from build123d import *

# Parameters (mm, degrees)
SKETCH2_R             = 6.35
BOSS_EXTRUDE1_DEPTH   = 19.05
BOSS_EXTRUDE1_2_DEPTH = 19.05
SKETCH3_W             = 139.7
SKETCH3_H             = 31.75
BOSS_EXTRUDE2_DEPTH   = 6.35
BOSS_EXTRUDE3_REACH   = 75.737
SKETCH9_W             = 133.75
SKETCH9_H             = 25.8
CUT_EXTRUDE1_DEPTH    = 3.175
CHAMFER2_SIZE         = 1.5875
HOLE1_D               = 5.715
HOLE1_DEPTH           = 12.7
HOLE1_CBORE_D         = 6.604
HOLE1_CBORE_DEPTH     = 0.6858


with BuildPart() as part:
    # Sketch2 → Boss-Extrude1 (new body)
    with BuildSketch(Plane(origin=(0, 0, 0), x_dir=(1, 0, 0), z_dir=(0, 1, 0))):
        with Locations(Location((-50.8, 0, 0), (0, 0, 90))):
            Circle(SKETCH2_R)
    extrude(amount=BOSS_EXTRUDE1_DEPTH)



with BuildPart() as body_2:
    # Sketch2 → Boss-Extrude1 2 (new body)
    with BuildSketch(Plane(origin=(0, 0, 0), x_dir=(1, 0, 0), z_dir=(0, 1, 0))):
        with Locations(Location((50.8, 0, 0), (0, 0, 90))):
            Circle(SKETCH2_R)
    extrude(amount=BOSS_EXTRUDE1_2_DEPTH)


with BuildPart() as part_1:
    add(part.part)

    add(body_2.part)  # Boss-Extrude2 merges body 2
    # Sketch3 → Boss-Extrude2 (add)
    with BuildSketch(Plane(origin=(0, 5.650833475, 8.701520484), x_dir=(-1, 0, 0), z_dir=(0, 0.5446390350150281, 0.8386705679454234))):
        with Locations((0, -15.976674319)):
            Rectangle(SKETCH3_W, SKETCH3_H)
    extrude(amount=BOSS_EXTRUDE2_DEPTH)

    # Sketch8 → Boss-Extrude3 (add, up to next)
    with BuildSketch(Plane(origin=(0, 19.05, 0), x_dir=(1, 0, 0), z_dir=(0, 1, 0)), mode=Mode.PRIVATE) as boss_extrude3_sk1:
        with BuildLine():
            Line((44.45, 0), (57.15, 0))
            ThreePointArc((57.15, 0), (50.8, 6.35), (44.45, 0))
        make_face()
    boss_extrude3_tool1 = extrude(boss_extrude3_sk1.sketch, amount=BOSS_EXTRUDE3_REACH, mode=Mode.PRIVATE) - part_1.part
    # Sketch8 → Boss-Extrude3 (add, up to next)
    with BuildSketch(Plane(origin=(0, 19.05, 0), x_dir=(1, 0, 0), z_dir=(0, 1, 0)), mode=Mode.PRIVATE) as boss_extrude3_sk2:
        with BuildLine():
            ThreePointArc((-44.45, 0), (-50.8, 6.35), (-57.15, 0))
            Line((-57.15, 0), (-44.45, 0))
        make_face()
    boss_extrude3_tool2 = extrude(boss_extrude3_sk2.sketch, amount=BOSS_EXTRUDE3_REACH, mode=Mode.PRIVATE) - part_1.part
    add(boss_extrude3_tool1.solids().sort_by_distance((50.8, 19.05, -2.695024))[0])
    add(boss_extrude3_tool2.solids().sort_by_distance((-50.8, 19.05, -2.695024))[0])

    # Sketch9 → Cut-Extrude1 (cut)
    with BuildSketch(Plane(origin=(0, 9.109291347, 14.02707859), x_dir=(1, 0, 0), z_dir=(0, 0.5446390350150282, 0.8386705679454234))):
        with Locations((0, 15.976674319)):
            Rectangle(SKETCH9_W, SKETCH9_H)
    extrude(amount=-CUT_EXTRUDE1_DEPTH, mode=Mode.SUBTRACT)

    # Chamfer2
    chamfer2_edges = [part_1.edges().sort_by_distance(p)[0] for p in [
        (69.85, 19.05, 0),
        (0, 5.736104734, 8.646144681),
        (0, 32.363895266, -8.646144681),
        (69.85, 34.093124202, -5.983365628),
        (-69.85, 19.05, 0),
        (-69.85, 34.093124202, -5.983365628),
        (0, 9.194562606, 13.971702787),
        (-69.85, 7.46533367, 11.308923734),
        (69.85, 22.508457872, 5.325558106),
        (69.85, 7.46533367, 11.308923734),
        (0, 35.822353138, -3.320586574),
        (-69.85, 22.508457872, 5.325558106),
    ]]
    chamfer(chamfer2_edges, length=CHAMFER2_SIZE)

    # Hole1
    with Locations(Plane(origin=(-50.8, 0, 0), x_dir=(0, 0, -1), z_dir=(0, -1, 0))):
        with Locations((0, 0), (0, 101.6)):
            CounterBoreHole(HOLE1_D / 2, HOLE1_CBORE_D / 2, HOLE1_CBORE_DEPTH, depth=HOLE1_DEPTH)


solid = part_1.part
The model under review builds one solid part; all positions refer to its coordinate system, in mm. A direction names the side the tool comes from. Round coordinates to 2 decimals unless told otherwise and drop trailing zeros. Order: outer loops, then holes, each group sorted by start corner. A loop starts at its lowest first (then second) coordinate and runs counter-clockwise, first axis right, second up. Notation, with made-up numbers: (-31.75, -11) -> (-4.75, -11) arc R24 ccw to (-4.75, 2) -> close; hole circle Ø9 at (-3, -24.75). An arc over 180 degrees is marked (long way). Return JSON: item names as keys, results as strings.
1. For L1, parallel to X at y = 0.25, z = 0; L2, parallel to X at y = 7.25, z = 0; L3, parallel to X at y = 28, z = 1.25 (3 decimals), list the stretches that pass through material, from the lowest coordinate up. Write a range as [from, to].
Answer block:
{"L1": "x = [-57.15, -54.1], [-47.5, -44.45], [44.45, 47.5], [54.1, 57.15]", "L2": "x = [-57.15, -53.66], [-47.94, -44.45], [44.45, 47.94], [53.66, 57.15]", "L3": "x = [-68.69, -66.875], [66.875, 68.69]"}
2. The part is to be moulded in two halves that separate along X. For faces 1 (the face through (-69.85, 21, 3)), 2 (the face through (0.956, 9.443, 12.877)), 3 (the face through (51, 12.7, 0)), say which applies: +X half, -X half, draft (parallel to the pull), parting line (faces both ways), or undercut.
Answer block:
{"face 1": "-X half", "face 2": "draft", "face 3": "undercut"}
3. Insertion check: P1, Ø3, axis at x = -0.5, z = 3.5, coming from the -Y side; P2, Ø1.5, axis at x = 25, z = -2, coming from the +Y side; P3, Ø3.5, axis at x = 50.8, z = 0, coming from the +Y side. Each pin has a flat end and moves straight along its axis. Give the tip position at first contact, or say it passes through.
Answer block:
{"P1": "stops at y = 11.35", "P2": "stops at y = 34.55", "P3": "stops at y = 33.4"}
4. Take a section at C-C (x = -50.8). Write out the cut boundary in (y, z), then the cut area to 3 significant figures.
Answer block:
{"outline": "(0, -6.35) -> (28.83, -6.35) -> (31.03, -7.78) -> (33.23, -7.31) -> (34.96, -4.65) -> (34.49, -2.46) -> (33.33, -1.7) -> (31.6, -4.36) -> (9.96, 9.69) -> (11.69, 12.35) -> (10.53, 13.11) -> (8.33, 12.64) -> (6.6, 9.98) -> (7.07, 7.78) -> (9.27, 6.35) -> (0, 6.35) -> (0, 3.3) -> (0.69, 3.3) -> (0.69, 2.86) -> (12.7, 2.86) -> (12.7, -2.86) -> (0.69, -2.86) -> (0.69, -3.3) -> (0, -3.3) -> close", "area": "283 mm²"}
5. Take a section at A-A (x = -32). Write out the cut boundary in (y, z), then the cut area to 3 significant figures.
Answer block:
{"outline": "(6.6, 9.98) -> (7.07, 7.78) -> (31.03, -7.78) -> (33.23, -7.31) -> (34.96, -4.65) -> (34.49, -2.46) -> (33.33, -1.7) -> (31.6, -4.36) -> (9.96, 9.69) -> (11.69, 12.35) -> (10.53, 13.11) -> (8.33, 12.64) -> close", "area": "115 mm²"}
6. For faces 4 (the face through (-0.936, 32.475, -3.013)), 5 (the face through (-69.045, 22.25, 4.56)), 6 (the face through (-47.526, 0.338, 0.43)), list the 3-axis set-ups (+Z, -Z, +X, -X, +Y, -Y) from which the entire face can be reached by the end or side of a thin tool; tool diameter is ignored.
Answer block:
{"face 4": "+Z", "face 5": "+Z, -X, +Y", "face 6": "-Y"}
